Autodesk Inventor part; units mm, degrees
ref_plane "YZ Plane" through (0, 0, 0) normal (1, 0, 0) x (0, 1, 0)
ref_plane "XZ Plane" through (0, 0, 0) normal (0, 1, 0) x (-1, 0, 0)
ref_plane "XY Plane" through (0, 0, 0) normal (0, 0, 1) x (1, 0, 0)
sketch "Sketch1" plane through (0, 0, 0) normal (0, 0, 1) x (1, 0, 0)
  line L0 (0, 0) -> (6.5, 0)
  line L1 (6.5, 0) -> (6.5, 5.13)
  line L2 (6.5, 5.13) -> (11.99, 5.13)
  line L3 (11.99, 5.13) -> (11.99, 13.25)
  line L4 (11.99, 13.25) -> (6.5, 13.25)
  line L5 (6.5, 13.25) -> (6.5, 18.38)
  line L6 (6.5, 18.38) -> (4, 18.38)
  line L7 (4, 18.38) -> (4, 68.95)
  line L8 (4, 68.95) -> (0, 68.95)
  line L9 (0, 68.95) -> (0, 0)
  dimension "d0" = 4
  dimension "d2" = 68.95
  dimension "d3" = 8.12
  dimension "d4" = 5.13
  dimension "d5" = 5.13
  dimension "d6" = 11.99
  dimension "d7" = 6.5
revolve "Revolution1" add sketch "Sketch1" angle 360 about axis through (0, 68.95, 0) along (0, -1, 0)
thread "Thread1"
properties part number "rod and bearing" material "Stainless Steel"
Read the model definition and answer for the solid it produces. Units are mm, in the model's axes. A direction names the side the tool comes from. Round coordinates to 2 decimals unless told otherwise and drop trailing zeros. Write each loop counter-clockwise with the first axis right and the second up, starting at its lowest first coordinate (ties: lowest second). Pieces come first, ordered by that corner, then holes.
1. Which of the six approach directions +Z, -Z, +X, -X, +Y, -Y give full straight-line access (tool end or side, diameter ignored) to faces 1 (the face through (0, 0, 0)), 2 (the face through (-5.158, 2.601, 3.955)), 3 (the face through (5, 13.25, -5))?
2. The part is cut by section A-A, the plane z = 0. Determine the outline of the cut face in (x, y).
3. Straight lines are drawn through the part: L1, parallel to Y at x = 7.25, z = -4.25; L2, parallel to Y at x = 1.25, z = -4.25; L3, parallel to X at y = 26.5, z = -2. For each, find the intervals that lie inside material, in ascending order.
4. The part is cut by section B-B, the plane x = 0. Determine the outline of the cut face in (y, z).
5. The part is cut by section C-C, the plane y = 31.5. Determine the outline of the cut face in (x, z), then the cut area to 3 significant figures.
6. Given pin 1 Ø8 at (y, z) = (59.5, -2) entering from +X; pin 2 Ø1.5 at (x, y) = (1.5, 59) entering from +Z; pin 3 Ø1.5 at (x, y) = (-2.5, 30) entering from +Z, each flat-ended and moving along its own axis, determine where each tip first touches the part or whether it passes through.
7. The part is cut by section D-D, the plane z = -5. Determine the outline of the cut face in (x, y).
Values:
1. face 1: +Z, -Z, +X, -X, -Y
1. face 2: -Y
1. face 3: +Y
2. outline: (-11.99, 5.13) - (-6.5, 5.13) - (-6.5, 0) - (6.5, 0) - (6.5, 5.13) - (11.99, 5.13) - (11.99, 13.25) - (6.5, 13.25) - (6.5, 18.38) - (4, 18.38) - (4, 68.95) - (-4, 68.95) - (-4, 18.38) - (-6.5, 18.38) - (-6.5, 13.25) - (-11.99, 13.25) - close
3. L1: y = 5.13 to 13.25
3. L2: y = 0 to 18.38
3. L3: x = -3.46 to 3.46
4. outline: (0, -6.5) - (5.13, -6.5) - (5.13, -11.99) - (13.25, -11.99) - (13.25, -6.5) - (18.38, -6.5) - (18.38, -4) - (68.95, -4) - (68.95, 4) - (18.38, 4) - (18.38, 6.5) - (13.25, 6.5) - (13.25, 11.99) - (5.13, 11.99) - (5.13, 6.5) - (0, 6.5) - close
5. outline: circle Ø8 at (0, 0)
5. area: 50.3 mm2
6. pin 1: stops at x = 4
6. pin 2: stops at z = 3.93
6. pin 3: stops at z = 3.6
7. outline: (-10.9, 5.13) - (-4.15, 5.13) - (-4.15, 0) - (4.15, 0) - (4.15, 5.13) - (10.9, 5.13) - (10.9, 13.25) - (4.15, 13.25) - (4.15, 18.38) - (-4.15, 18.38) - (-4.15, 13.25) - (-10.9, 13.25) - close
